```python
from build123d import *

# Parameters (mm, degrees)
CROQUIS1_W              = 30
CROQUIS1_H              = 35
CROQUIS1_R              = 1.5
SALIENTE_EXTRUIR1_DEPTH = 20
CROQUIS2_W              = 10
CROQUIS2_H              = 4
CORTAR_EXTRUIR1_DEPTH   = 41
CORTAR_EXTRUIR2_DEPTH   = 8
CORTAR_EXTRUIR3_DEPTH   = 8
CROQUIS6_W              = 30
CROQUIS6_H              = 11
SALIENTE_EXTRUIR2_DEPTH = 10
CORTAR_EXTRUIR4_START   = -30
CROQUIS7_W              = 45
CROQUIS7_H              = 6
CORTAR_EXTRUIR4_DEPTH   = 30
CORTAR_EXTRUIR5_REACH   = 52.249
CROQUIS8_W              = 4
CROQUIS8_H              = 5
CORTAR_EXTRUIR6_START   = -30
CROQUIS9_W              = 12.7
CROQUIS9_H              = 5
CORTAR_EXTRUIR6_DEPTH   = 30
REDONDEO1_R             = 3


with BuildPart() as part:
    # Croquis1 → Saliente-Extruir1 (new body)
    with BuildSketch(Plane(origin=(0, 0, 0), x_dir=(1, 0, 0), z_dir=(0, 1, 0))):
        with Locations((15, 17.5)):
            Rectangle(CROQUIS1_W, CROQUIS1_H)
        with Locations(Location((25, 30, 0), (0, 0, 270))):
            Circle(CROQUIS1_R, mode=Mode.SUBTRACT)
        with Locations(Location((5, 30, 0), (0, 0, 270))):
            Circle(CROQUIS1_R, mode=Mode.SUBTRACT)
        with Locations(Location((7.5, 5, 0), (0, 0, 270))):
            Circle(CROQUIS1_R, mode=Mode.SUBTRACT)
        with Locations(Location((22.5, 5, 0), (0, 0, 270))):
            Circle(CROQUIS1_R, mode=Mode.SUBTRACT)
    extrude(amount=SALIENTE_EXTRUIR1_DEPTH)

    # Croquis2 → Cortar-Extruir1 (cut)
    with BuildSketch(Plane(origin=(30, 0, 0), x_dir=(0, 0, -1), z_dir=(1, 0, 0))):
        with Locations((30, 13)):
            Rectangle(CROQUIS2_W, CROQUIS2_H)
    extrude(amount=-CORTAR_EXTRUIR1_DEPTH, mode=Mode.SUBTRACT)

    # Croquis3 → Cortar-Extruir2 (cut)
    with BuildSketch(Plane.XZ):
        Polygon((5, -33.117691454), (7.7, -31.558845727), (7.7, -28.441154273), (5, -26.882308546), (2.3, -28.441154273), (2.3, -31.558845727), align=None)
        Polygon((25, -33.117691454), (27.7, -31.558845727), (27.7, -28.441154273), (25, -26.882308546), (22.3, -28.441154273), (22.3, -31.558845727), align=None)
    extrude(amount=-CORTAR_EXTRUIR2_DEPTH, mode=Mode.SUBTRACT)

    # Croquis4 → Cortar-Extruir3 (cut)
    with BuildSketch(Plane.XZ):
        Polygon((7.5, -8.117691454), (10.2, -6.558845727), (10.2, -3.441154273), (7.5, -1.882308546), (4.8, -3.441154273), (4.8, -6.558845727), align=None)
        Polygon((22.5, -8.117691454), (25.2, -6.558845727), (25.2, -3.441154273), (22.5, -1.882308546), (19.8, -3.441154273), (19.8, -6.558845727), align=None)
    extrude(amount=-CORTAR_EXTRUIR3_DEPTH, mode=Mode.SUBTRACT)

    # Croquis6 → Saliente-Extruir2 (add)
    with BuildSketch(Plane(origin=(0, 0, -35), x_dir=(-1, 0, 0), z_dir=(0, 0, -1))):
        with Locations((-15, 5.5)):
            Rectangle(CROQUIS6_W, CROQUIS6_H)
    extrude(amount=SALIENTE_EXTRUIR2_DEPTH)

    # Croquis7 → Cortar-Extruir4 (cut)
    with BuildSketch(Plane.ZY.offset(CORTAR_EXTRUIR4_START)):
        with Locations((-22.5, 3)):
            Rectangle(CROQUIS7_W, CROQUIS7_H)
    extrude(amount=CORTAR_EXTRUIR4_DEPTH, mode=Mode.SUBTRACT)

    # Cortar-Extruir5: up to this face of the body (flat: up to its plane)
    cortar_extruir5_end = Plane(part.part.faces().sort_by_distance((15, 13, 0))[0])
    # Croquis8 → Cortar-Extruir5 (cut, up to the picked face)
    with BuildSketch(Plane(origin=(0, 0, -35), x_dir=(-1, 0, 0), z_dir=(0, 0, -1)), mode=Mode.PRIVATE) as cortar_extruir5_sk1:
        with Locations((-15, 17.5)):
            Rectangle(CROQUIS8_W, CROQUIS8_H)
    cortar_extruir5_tool1 = split(extrude(cortar_extruir5_sk1.sketch, amount=-CORTAR_EXTRUIR5_REACH, mode=Mode.PRIVATE), bisect_by=cortar_extruir5_end, keep=Keep.BOTH, mode=Mode.PRIVATE)
    add(cortar_extruir5_tool1.solids().sort_by(Axis((15, 17.5, -35), (0, 0, 1)))[0], mode=Mode.SUBTRACT)

    # Croquis9 → Cortar-Extruir6 (cut)
    with BuildSketch(Plane.ZY.offset(CORTAR_EXTRUIR6_START)):
        with Locations((-6.35, 17.5)):
            Rectangle(CROQUIS9_W, CROQUIS9_H)
    extrude(amount=CORTAR_EXTRUIR6_DEPTH, mode=Mode.SUBTRACT)

    # Redondeo1
    redondeo1_edges = [part.edges().sort_by_distance(p)[0] for p in [
        (30, 10.5, 0),
        (0, 10.5, 0),
    ]]
    fillet(redondeo1_edges, radius=REDONDEO1_R)


solid = part.part
```
The model under review builds one solid part; all positions refer to its coordinate system, in mm. A direction names the side the tool comes from. Round coordinates to 2 decimals unless told otherwise and drop trailing zeros. Loops run counter-clockwise (first coordinate to the right, second up) from the corner with the lowest first, then second, coordinate; pieces in that order, holes last. Notation, with made-up numbers: (-2.75, 84.25) - (23.25, 84.25) arc R29 cw to (23.25, 122.25) - close; hole circle Ø8 at (29, -10.75). An arc over 180 degrees is marked (long way). Use a Markdown table: item, result. Add a question column.
Q1. Add section C-C (z = -14.5). State the section outline as (x, y) points, plus the area to 3 significant figures.
Q2. Add section B-B (y = 10.5). State the section outline as (x, z) points, plus the area to 3 significant figures.
Q3. The part is to be moulded in two halves that separate along Z. For faces 1 (the face through (15, 13, -25)), 2 (the face through (29.14, 10.56, -0.9)), 3 (the face through (24, 8, -6)), say which applies: pulls with the +Z half, pulls with the -Z half, needs draft (parallel to the pull), parting line crosses it, or undercut.
Q4. Add section D-D (x = 24.5). State the section outline as (y, z) points, plus the area to 3 significant figures.
Q5. For probe 1 along X at (y, z) = (12.5, -5); probe 2 along X at (y, z) = (18.6, -30); probe 3 along X at (y, z) = (16.5, -19.5), list the stretches that pass through material, from the lowest coordinate up.
Q6. Add section A-A (y = 16.25). State the section outline as (x, z) points.
Q7. Machinability: for faces 4 (the face through (27.7, 7, -30)), 5 (the face through (6, 17, -35)), 6 (the face through (15, 11, -35)), which of the approach directions +Z, -Z, +X, -X, +Y, -Y give a long, thin tool a straight path to every point of the face, cutting with its end or side? Answer none if there is none.
Q8. Insertion check: pin 1 Ø5 at (y, z) = (13.5, -36.5) entering from -X; pin 2 Ø2.5 at (x, z) = (22.5, -5) entering from +Y; pin 3 Ø2.5 at (x, y) = (5.5, 18) entering from +Z; pin 4 Ø2.5 at (x, y) = (6, 17.5) entering from -Z. Each pin has a flat end and moves straight along its axis. Give the tip position at first contact, or say it passes through.
Worked answers:
| question | item | result |
|---|---|---|
| 1 | outline | (0, 6) - (30, 6) - (30, 20) - (17, 20) - (17, 15) - (13, 15) - (13, 20) - (0, 20) - close |
| 1 | area | 400 mm² |
| 2 | outline | (0, -45) - (30, -45) - (30, -3) arc R3 ccw to (27, 0) - (3, 0) arc R3 ccw to (0, -3) - close; hole circle Ø3 at (5, -30); hole circle Ø3 at (7.5, -5); hole circle Ø3 at (22.5, -5); hole circle Ø3 at (25, -30) |
| 2 | area | 1,320 mm² |
| 3 | face 1 | pulls with the -Z half |
| 3 | face 2 | pulls with the +Z half |
| 3 | face 3 | undercut |
| 4 | outline | (6, -45) - (11, -45) - (11, -31.41) - (8, -31.41) - (8, -32.83) - (6, -32.83) - close; (6, -27.17) - (8, -27.17) - (8, -28.59) - (11, -28.59) - (11, -25) - (15, -25) - (15, -28.59) - (20, -28.59) - (20, -12.7) - (15, -12.7) - (15, 0) - (6, 0) - (6, -3.04) - (8, -3.04) - (8, -6.96) - (6, -6.96) - close; (15, -35) - (20, -35) - (20, -31.41) - (15, -31.41) - close |
| 4 | area | 395 mm² |
| 5 | probe 1 | 0 to 6, 9 to 21, 24 to 30 |
| 5 | probe 2 | 0 to 3.5, 6.5 to 13, 17 to 23.5, 26.5 to 30 |
| 5 | probe 3 | 0 to 13, 17 to 30 |
| 6 | outline | (0, -35) - (13, -35) - (13, -12.7) - (0, -12.7) - close; (17, -35) - (30, -35) - (30, -12.7) - (17, -12.7) - close; hole circle Ø3 at (5, -30); hole circle Ø3 at (25, -30) |
| 7 | face 4 | -Y |
| 7 | face 5 | -Z, +X, -X, +Y |
| 7 | face 6 | -Z, +X, -X |
| 8 | pin 1 | x = 0 |
| 8 | pin 2 | through |
| 8 | pin 3 | z = -12.7 |
| 8 | pin 4 | z = -35 |
